Work out the finished part from the listing and answer in its coordinate system (mm). A direction names the side the tool comes from. Give positions to 0.01 mm unless a question says otherwise; leave off trailing zeros. Loops run counter-clockwise (first coordinate to the right, second up) from the corner with the lowest first, then second, coordinate; pieces in that order, holes last. Notation, with made-up numbers: (-15.75, 68.25) - (27.25, 68.25) arc R18 cw to (27.25, 96.25) - close; hole circle Ø11 at (55, 46). An arc over 180 degrees is marked (long way). Use CSV: the item, a comma, the result in double quotes.
from build123d import *

# Parameters (mm, degrees)
SKETCH1_R           = 3.175
EXTRUDE1_DEPTH      = 11.1125
SKETCH2_R           = 4.826
EXTRUDE2_DEPTH      = 2.54
CHAMFER1_SIZE       = 0.508
SKETCH3_R           = 1.190625
EXTRUDE3_DEPTH      = 5.826
EXTRUDE3_DEPTH_BACK = 5.826
CHAMFER2_SIZE       = 0.3175


with BuildPart() as part:
    # Sketch1 → Extrude1 (new body, symmetric)
    with BuildSketch(Plane.XY):
        Circle(SKETCH1_R)
    extrude(amount=EXTRUDE1_DEPTH, both=True)

    # Sketch2 → Extrude2 (add)
    with BuildSketch(Plane.XY.offset(11.1125)):
        Circle(SKETCH2_R)
    extrude(amount=EXTRUDE2_DEPTH)

    # Chamfer1
    chamfer1_edges = [part.edges().sort_by_distance(p)[0] for p in [
        (-4.826, 0, 13.6525),
    ]]
    chamfer(chamfer1_edges, length=CHAMFER1_SIZE)

    # Sketch3 → Extrude3 (cut, two sides)
    with BuildSketch(Plane(origin=(0, 0, 0), x_dir=(0, 0, -1), z_dir=(1, 0, 0))) as extrude3_sk:
        with Locations((7.540625, 0)):
            Circle(SKETCH3_R)
    extrude(amount=EXTRUDE3_DEPTH, mode=Mode.SUBTRACT)
    extrude(extrude3_sk.sketch, amount=-EXTRUDE3_DEPTH_BACK, mode=Mode.SUBTRACT)

    # Chamfer2
    chamfer2_edges = [part.edges().sort_by_distance(p)[0] for p in [
        (-3.175, 0, -11.1125),
    ]]
    chamfer(chamfer2_edges, length=CHAMFER2_SIZE)


solid = part.part
Item 1: Given P1, Ø1, axis at x = -3, z = 2, coming from the -Y side; P2, Ø1.5, axis at y = 3.5, z = 6.5, coming from the +X side; P3, Ø4, axis at y = 0, z = -7.54, coming from the -X side (3 decimals), each flat-ended and moving along its own axis, determine where each tip first touches the part or whether it passes through.
Determined:
P1,"stops at y = -1.96"
P2,"stops at x = 1.59"
P3,"stops at x = -3.175"
Item 2: A cutting plane is placed at B-B on z = -7.25. Determine the outline of the cut face in (x, y) (3 decimals), and give its area (3 significant figures).
Determined:
outline,"(-2.958, -1.155) arc R3.175 ccw to (2.958, -1.155) - close; (-2.958, 1.155) - (2.958, 1.155) arc R3.175 ccw to start"
area,"17.3 mm²"
Item 3: For faces 1 (the flat face through (-1.14, -3.15, 11.112)), 2 (the cylindrical face through (-3.83, -2.937, 12.114)), determine the directions among +Z, -Z, +X, -X, +Y, -Y from which every point of the face is accessible in a straight line to the end or side of a thin tool.
Determined:
face 1,"-Z"
face 2,"+Z, -Z"
Item 4: Find the intervals of material crossed by line 1 (Z direction, x = 1.9, y = 0); line 2 (Z direction, x = -3, y = -1.75); line 3 (X direction, y = 0, z = -4.5) (3 decimals), in increasing order.
Determined:
line 1,"z = -11.11 to -8.73, -6.35 to 13.65"
line 2,"z = 11.11 to 13.65"
line 3,"x = -3.175 to 3.175"
Item 5: A cutting plane is placed at C-C on z = 8. Determine the outline of the cut face in (x, y) (3 decimals).
Determined:
outline,"circle Ø6.35 at (0, 0)"
